from build123d import *

# Parameters (mm, degrees)
F0_W      = 23
F0_H      = 22
F1_DEPTH  = 6
F2_W      = 33
F2_H      = 2
F3_DEPTH  = 12
F4_R      = 6
F5_DEPTH  = 4
F7_DEPTH  = 4
F8_R      = 2.5
F9_DEPTH  = 3
F11_DEPTH = 18.001
F13_DEPTH = 18.001


with BuildPart() as f1:
    # F0 (on Front) → F1 (new body, symmetric)
    with BuildSketch(Plane.XZ):
        with Locations((0, 11)):
            Rectangle(F0_W, F0_H)
    extrude(amount=F1_DEPTH, both=True)

    # F2 (on face) → F3 (join)
    with BuildSketch(Plane.XZ.offset(6)):
        with Locations((0, 17)):
            Rectangle(F2_W, F2_H)
    extrude(amount=-F3_DEPTH)

    # F4 (on face) → F5 (join)
    with BuildSketch(Plane.XY.offset(22)):
        with Locations((-5.5, 0)):
            Circle(F4_R)
    extrude(amount=F5_DEPTH)

    # F6 (on face) → F7 (join)
    with BuildSketch(Plane.XY.offset(22)):
        with BuildLine():
            Line((-2, -2.5), (1, -2.5))
            ThreePointArc((1, -2.5), (3.5, 0), (1, 2.5))
            Line((1, 2.5), (-2, 2.5))
            Line((-2, 2.5), (-2, -2.5))
        make_face()
    extrude(amount=F7_DEPTH)

    # F8 (on face) → F9 (join)
    with BuildSketch(Plane.XY.offset(26)):
        with Locations((-5.5, 0)):
            Circle(F8_R)
    extrude(amount=F9_DEPTH)

    # F10 (on face) → F11 (cut, through all)
    with BuildSketch(Plane.XY.offset(18)):
        with BuildLine():
            Line((16.745644, 0.5), (16.245644, 0.5))
            ThreePointArc((16.245644, 0.5), (13.85, 0), (16.245644, -0.5))
            Line((16.245644, -0.5), (16.745644, -0.5))
            Line((16.745644, -0.5), (16.745644, 0.5))
        make_face()
    extrude(amount=-F11_DEPTH, mode=Mode.SUBTRACT)

    # F12 (on face) → F13 (cut, through all)
    with BuildSketch(Plane.XY.offset(18)):
        with BuildLine():
            Line((-16.934745, -0.5), (-16.245644, -0.5))
            ThreePointArc((-16.245644, -0.5), (-13.85, 0), (-16.245644, 0.5))
            Line((-16.245644, 0.5), (-16.934745, 0.5))
            Line((-16.934745, 0.5), (-16.934745, -0.5))
        make_face()
    extrude(amount=-F13_DEPTH, mode=Mode.SUBTRACT)


solid = f1.part
Geometry check sheet. Reference: the model listing, model coordinates, mm. A direction names the side the tool comes from. Give positions to 0.01 mm unless a question says otherwise; leave off trailing zeros. Loops run counter-clockwise (first coordinate to the right, second up) from the corner with the lowest first, then second, coordinate; pieces in that order, holes last.
(1) Depth check by flat-ended pin: pin 1 Ø2 at (y, z) = (-0.5, 12) entering from -X; pin 2 Ø0.5 at (x, z) = (0.5, 25) entering from +Y; pin 3 Ø6 at (x, y) = (3, -3) entering from +Z; pin 4 Ø1.5 at (x, z) = (-13, 15.5) entering from +Y. Enter the tip coordinate at first touch or a pass-through.
From the geometry:
pin 1: stops at x = -11.5
pin 2: stops at y = 2.5
pin 3: stops at z = 26
pin 4: stops at y = 6
(2) Section check B-B on y = -3.25. Record the cut outline in (x, z).
From the geometry:
outline: (-16.5, 16) - (-11.5, 16) - (-11.5, 0) - (11.5, 0) - (11.5, 16) - (16.5, 16) - (16.5, 18) - (11.5, 18) - (11.5, 22) - (-0.46, 22) - (-0.46, 26) - (-10.54, 26) - (-10.54, 22) - (-11.5, 22) - (-11.5, 18) - (-16.5, 18) - close
(3) Section check D-D on z = 19.25. Record the cut outline in (x, y), then the cut area to 3 significant figures.
From the geometry:
outline: (-11.5, -6) - (11.5, -6) - (11.5, 6) - (-11.5, 6) - close
area: 276 mm2
(4) Section check C-C on x = -6.5. Record the cut outline in (y, z), then the cut area to 3 significant figures.
From the geometry:
outline: (-6, 0) - (6, 0) - (6, 22) - (5.92, 22) - (5.92, 26) - (2.29, 26) - (2.29, 29) - (-2.29, 29) - (-2.29, 26) - (-5.92, 26) - (-5.92, 22) - (-6, 22) - close
area: 325 mm2
(5) Release check for a two-part mould opening along X. For faces 1 (the flat face through (11.5, 0, 8)), 2 (the cylindrical face through (-13.85, -0.05, 17.01)), 3 (the cylindrical face through (-11.496, 0.228, 23.972)), 4 (the flat face through (13, 0, 16)) record: released by +X, released by -X, zero draft, split by the parting line, or undercut.
From the geometry:
face 1: released by +X
face 2: undercut
face 3: split by the parting line
face 4: zero draft
(6) Section check A-A on x = 15.1. Record the cut outline in (y, z).
From the geometry:
outline: (-6, 16) - (-1.25, 16) - (-1.25, 18) - (-6, 18) - close; (1.25, 16) - (6, 16) - (6, 18) - (1.25, 18) - close
(7) Thickness scan on L1, parallel to Y at x = -15.1, z = 17.55; L2, parallel to Z at x = -8, y = -3.5; L3, parallel to X at y = 0, z = 16.5. Record the ranges inside material, lowest first.
From the geometry:
L1: y = -6 to -1.25, 1.25 to 6
L2: z = 0 to 26
L3: x = -13.85 to 13.85
(8) Set-up check for faces 5 (the flat face through (5, 0, 22)), 6 (the flat face through (-13, 0, 16)), 7 (the cylindrical face through (-3.115, 0.751, 27.479)), 8 (the flat face through (11.5, 0, 20)): record each of +Z, -Z, +X, -X, +Y, -Y from which the full face is reachable in a straight line by a thin tool's end or side.
From the geometry:
face 5: +Z, +X
face 6: -Z, -X, +Y, -Y
face 7: +Z
face 8: +Z, +X, +Y, -Y
